```python
from build123d import *

# Parameters (mm, degrees)
F1_DEPTH = 38.1
F2_R     = 25.4
F3_SIZE  = 25.4


with BuildPart() as f1:
    # F0 (on Front) → F1 (new body)
    with BuildSketch(Plane.XZ):
        Polygon((-659.911358, 0), (0, 0), (-659.911358, 381), align=None)
        Polygon((-659.911358, 381), (0, 0), (0, 381), align=None)
    extrude(amount=F1_DEPTH)

    # F2
    f2_edges = [f1.edges().sort_by_distance(p)[0] for p in [
        (-659.911358, -19.05, 381),
        (0, -19.05, 381),
        (0, -19.05, 0),
        (-659.911358, -19.05, 0),
    ]]
    fillet(f2_edges, radius=F2_R)

    # F3
    f3_edges = [f1.edges().sort_by_distance(p)[0] for p in [
        (-659.911358, 0, 190.5),
        (-652.47187, 0, 373.560512),
        (-652.47187, 0, 7.439488),
        (-329.955679, 0, 381),
        (-329.955679, 0, 0),
        (-7.439488, 0, 373.560512),
        (-7.439488, 0, 7.439488),
        (0, 0, 190.5),
    ]]
    chamfer(f3_edges, length=F3_SIZE)


solid = f1.part
```
Read the model definition and answer for the solid it produces. Units are mm, in the model's axes. Coordinates: 2 decimals unless noted, no trailing zeros. Loops run counter-clockwise (first coordinate to the right, second up) from the corner with the lowest first, then second, coordinate; pieces in that order, holes last. Notation, with made-up numbers: (4.25, -30.75) -> (17.25, -30.75) arc R19 cw to (17.25, -26.75) -> close; hole circle Ø8 at (-7, 72.5). An arc over 180 degrees is marked (long way). Return JSON: item names as keys, results as strings.
Item 1: Flat-ended cylindrical pins translate along their axes: P1, Ø8, axis at y = -18, z = 317, coming from the -X side; P2, Ø12, axis at x = -131, y = -13, coming from the +Z side; P3, Ø2, axis at y = -16, z = 207.5, coming from the -X side. Find the tip coordinate at first contact, or state that the pin passes through.
Answers:
{"P1": "stops at x = -656.51", "P2": "stops at z = 374.6", "P3": "stops at x = -651.51"}
Item 2: Find the intervals of material crossed by probe 1 along Z at (x, y) = (-342.5, -11.5); probe 2 along Z at (x, y) = (-484, -5); probe 3 along X at (y, z) = (-23, 190.5), in increasing order.
Answers:
{"probe 1": "z = 13.9 to 367.1", "probe 2": "z = 20.4 to 360.6", "probe 3": "x = -657.51 to -2.4"}
Item 3: Find section B-B (z = 253). Determine the outline of the cut face in (x, y).
Answers:
{"outline": "(-659.91, -38.1) -> (0, -38.1) -> (0, -25.4) -> (-25.4, 0) -> (-634.51, 0) -> (-659.91, -25.4) -> close"}
Item 4: Find section A-A (x = -438). Determine the outline of the cut face in (y, z), plus the area to 3 significant figures.
Answers:
{"outline": "(-38.1, 0) -> (-25.4, 0) -> (0, 25.4) -> (0, 355.6) -> (-25.4, 381) -> (-38.1, 381) -> close", "area": "13,900 mm2"}
